Geometry: final body of the model. Coordinates: model frame, mm. A direction names the side the tool comes from. Give positions to 0.01 mm unless a question says otherwise; leave off trailing zeros. Write each loop counter-clockwise with the first axis right and the second up, starting at its lowest first coordinate (ties: lowest second). Pieces come first, ordered by that corner, then holes. Notation, with made-up numbers: M 87,88 L 98,88 A12 cw 98,101 Z; hole C -7,64.25 d2. An arc over 180 degrees is marked long. Use a Markdown table: item, result. Add a question column.
1) Set-up query: faces 4 (the flat face through (-1, 2.405, 3)), 5 (the flat face through (6.797, 6, 3)), 6 (the flat face through (5, 2.405, 3)). Return all of +Z, -Z, +X, -X, +Y, -Y with unobstructed straight access to the full face (end or side cutting, diameter ignored); none if empty.
2) Section C-C on x = 2.25. Return the cut outline in (y, z), then the cut area to 3 significant figures.
3) Section B-B on z = 2. Return the cut outline in (x, y).
4) Section A-A on x = 0. Return the cut outline in (y, z), then the cut area to 3 significant figures.
5) Draft query along Y for faces 1 (the flat face through (2, -0.595, 4)), 2 (the flat face through (0.29, 0.88, 3.97)), 3 (the flat face through (2, 5, 0)). Return one class per face: +Y half, -Y half, draft (parallel to the pull), parting line (faces both ways), or undercut.
6) Section D-D on y = 2.75. Return the cut outline in (x, z), then the cut area to 3 significant figures.
7) Pin query (flat end, axial travel): pin 1 (4 mm diameter, centred on x = 5.5, y = 9, fed in from +Z). Return the tip coordinate at first contact, or that it passes through.
8) Line query: line 1 (Y direction, x = -0.5, z = 1.5); line 2 (Z direction, x = 6, y = 7.75); line 3 (Y direction, x = -0.75, z = 4). Output: solid intervals per line, ascending.
```python
from build123d import *

# Parameters (mm, degrees)
BOSS_EXTRUDE1_DEPTH     = 10
CUT_EXTRUDE1_DEPTH      = 18.007618008
CUT_EXTRUDE1_DEPTH_BACK = 18.007618008


with BuildPart() as part:
    # Sketch2 → Boss-Extrude1 (new body)
    with BuildSketch(Plane.XY):
        Polygon((0.796949894, 2.404761905), (-2.203050106, 2.404761905), (-2.203050106, 10.404761905), (6.796949894, 10.404761905), (6.796949894, 2.404761905), (3.796949894, 2.404761905), (4.796949894, -0.595238095), (-0.203050106, -0.595238095), align=None)
    extrude(amount=BOSS_EXTRUDE1_DEPTH)

    # Sketch3 → Cut-Extrude1 (cut, two sides: drawn at the far end of the back side and taken through both)
    with BuildSketch(Plane(origin=(6.796949894, 0, 0), x_dir=(0, 0, -1), z_dir=(1, 0, 0)).offset(-CUT_EXTRUDE1_DEPTH_BACK)):
        Polygon((-3.5, 10.404761905), (-10, 10.404761905), (-10, 2.404761905), (-6.813708499, 2.404761905), align=None)
        Polygon((-6.813708499, 2.404761905), (-10, 2.404761905), (-10, -0.595238095), (-8.056349186, -0.595238095), align=None)
    extrude(amount=CUT_EXTRUDE1_DEPTH + CUT_EXTRUDE1_DEPTH_BACK, mode=Mode.SUBTRACT)


solid = part.part
```
Found:
| question | item | result |
|---|---|---|
| 1 | face 4 | +Z, -Z, -X |
| 1 | face 5 | +Z, -Z, +X, +Y, -Y |
| 1 | face 6 | +Z, -Z, +X |
| 2 | outline | M -0.6,0 L 10.4,0 L 10.4,3.5 L -0.6,8.06 Z |
| 2 | area | 63.6 mm² |
| 3 | outline | M -2.2,2.4 L 0.8,2.4 L -0.2,-0.6 L 4.8,-0.6 L 3.8,2.4 L 6.8,2.4 L 6.8,10.4 L -2.2,10.4 Z |
| 4 | outline | M -0.6,0 L 0.01,0 L 0.01,7.8 L -0.6,8.06 Z; M 2.4,0 L 10.4,0 L 10.4,3.5 L 2.4,6.81 Z |
| 4 | area | 46.1 mm² |
| 5 | face 1 | -Y half |
| 5 | face 2 | undercut |
| 5 | face 3 | draft |
| 6 | outline | M -2.2,0 L 6.8,0 L 6.8,6.67 L -2.2,6.67 Z |
| 6 | area | 60.0 mm² |
| 7 | pin 1 | z = 4.91 |
| 8 | line 1 | 2.4 to 10.4 |
| 8 | line 2 | 0 to 4.6 |
| 8 | line 3 | 2.4 to 9.2 |
